from build123d import *

# Parameters (mm, degrees)
CROQUIS1_R              = 18.39
SALIENTE_EXTRUIR1_DEPTH = 6
CROQUIS3_R              = 8.675
SALIENTE_EXTRUIR2_DEPTH = 11.6
CROQUIS4_R              = 4.05
CORTAR_EXTRUIR1_DEPTH   = 31.6


with BuildPart() as part:
    # Croquis1 → Saliente-Extruir1 (new, symmetric)
    with BuildSketch(Plane.XY):
        Circle(CROQUIS1_R)
    extrude(amount=SALIENTE_EXTRUIR1_DEPTH, both=True)

    # Croquis3 → Saliente-Extruir2 (add)
    with BuildSketch(Plane.XY.offset(6)):
        Circle(CROQUIS3_R)
    extrude(amount=SALIENTE_EXTRUIR2_DEPTH)

    # Croquis4 → Cortar-Extruir1 (cut)
    with BuildSketch(Plane.XY.offset(17.6)):
        Circle(CROQUIS4_R)
    extrude(amount=-CORTAR_EXTRUIR1_DEPTH, mode=Mode.SUBTRACT)


solid = part.part
Geometry check sheet. Reference: the model listing, model coordinates, mm. A direction names the side the tool comes from. Give positions to 0.01 mm unless a question says otherwise; leave off trailing zeros. Loops run counter-clockwise (first coordinate to the right, second up) from the corner with the lowest first, then second, coordinate; pieces in that order, holes last. Notation, with made-up numbers: (69.5, 59) -> (82.5, 59) arc R26 cw to (82.5, 82) -> close; hole circle Ø6 at (-5, -15.75). An arc over 180 degrees is marked (long way). Answer in a Markdown table with one row per item. Add a question column.
1) Gauge pin test, flat ends, axial feed: P1, Ø12, axis at x = 9.5, z = 3, coming from the -Y side; P2, Ø1.5, axis at x = -11, y = 1.5, coming from the +Z side; P3, Ø8, axis at x = 12, z = 2.5, coming from the -Y side; P4, Ø9.5, axis at x = 0, y = 0, coming from the -Z side. Record the tip position at first contact, or that the pin passes through.
2) Cross-section at D-D on y = 7.5. Record the boundary of the cut face in (x, z), and give its area (3 significant figures).
3) Set-up check for faces 4 (the face through (8.486, -16.315, 0.084)), 5 (the face through (8, -4, 6)): record each of +Z, -Z, +X, -X, +Y, -Y from which the full face is reachable in a straight line by a thin tool's end or side.
4) Cross-section at A-A on y = 0. Record the boundary of the cut face in (x, z) (3 decimals), and give its area (3 significant figures).
5) Draft check along Y on faces 1 (the face through (-1.13, 8.6, 11.72)), 2 (the face through (-0.878, -3.954, 5.965)), 3 (the face through (-0.3, 4.3, -6)). Enter one of: pulls with the +Y half, pulls with the -Y half, needs draft (parallel to the pull), parting line crosses it, or undercut.
6) Cross-section at C-C on z = -2.5. Record the boundary of the cut face in (x, y), and give its area (3 significant figures).
7) Material ranges on probe 1 along Y at (x, z) = (0, 11) (3 decimals); probe 2 along Y at (x, z) = (0, 3.75); probe 3 along Z at (x, y) = (-10.5, 2), recorded low to high. Write a range as from..to.
Outcome:
| question | item | result |
|---|---|---|
| 1 | P1 | stops at y = -18.05 |
| 1 | P2 | stops at z = 6 |
| 1 | P3 | stops at y = -16.56 |
| 1 | P4 | stops at z = -6 |
| 2 | outline | (-16.79, -6) -> (16.79, -6) -> (16.79, 6) -> (4.36, 6) -> (4.36, 17.6) -> (-4.36, 17.6) -> (-4.36, 6) -> (-16.79, 6) -> close |
| 2 | area | 504 mm^2 |
| 3 | face 4 | +Z, -Z |
| 3 | face 5 | +Z |
| 4 | outline | (-18.39, -6) -> (-4.05, -6) -> (-4.05, 17.6) -> (-8.675, 17.6) -> (-8.675, 6) -> (-18.39, 6) -> close; (4.05, -6) -> (18.39, -6) -> (18.39, 6) -> (8.675, 6) -> (8.675, 17.6) -> (4.05, 17.6) -> close |
| 4 | area | 451 mm^2 |
| 5 | face 1 | parting line crosses it |
| 5 | face 2 | undercut |
| 5 | face 3 | needs draft |
| 6 | outline | circle Ø36.78 at (0, 0); hole circle Ø8.1 at (0, 0) |
| 6 | area | 1,010 mm^2 |
| 7 | probe 1 | y = -8.675..-4.05, 4.05..8.675 |
| 7 | probe 2 | y = -18.39..-4.05, 4.05..18.39 |
| 7 | probe 3 | z = -6..6 |
